```python
from build123d import *

# Parameters (mm, degrees)
SKETCH1_W            = 40
SKETCH1_H            = 20
BOSS_EXTRUDE1_DEPTH  = 35.3
BOSS_EXTRUDE2_DEPTH  = 2
SKETCH3_R            = 6.458580866
BOSS_EXTRUDE3_DEPTH  = 1.5
SKETCH4_R            = 5.433415679
BOSS_EXTRUDE4_DEPTH  = 1.5
SKETCH5_R            = 2.875
BOSS_EXTRUDE5_DEPTH  = 4
SKETCH6_W            = 20
SKETCH6_H            = 2.5
BOSS_EXTRUDE6_DEPTH  = 6
CUT_EXTRUDE1_DEPTH   = 7
SKETCH8_W            = 20
SKETCH8_H            = 2.5
BOSS_EXTRUDE7_DEPTH  = 6
CUT_EXTRUDE2_DEPTH   = 7
SKETCH11_W           = 7
SKETCH11_H           = 4
BOSS_EXTRUDE8_DEPTH  = 6
SKETCH12_W           = 6.5
SKETCH12_H           = 3.5
CUT_EXTRUDE3_DEPTH   = 6
SKETCH13_W           = 6
SKETCH13_H           = 1.3
BOSS_EXTRUDE9_DEPTH  = 1.5
SKETCH14_W           = 6
SKETCH14_H           = 1.3
BOSS_EXTRUDE10_DEPTH = 1.5
CUT_EXTRUDE4_DEPTH   = 1.5
CUT_EXTRUDE5_DEPTH   = 1.5
SKETCH17_R           = 1.5
CUT_EXTRUDE6_DEPTH   = 4


with BuildPart() as part:
    # Sketch1 → Boss-Extrude1 (new body)
    with BuildSketch(Plane(origin=(0, 0, 0), x_dir=(1, 0, 0), z_dir=(0, 1, 0))):
        with Locations((20, 10)):
            Rectangle(SKETCH1_W, SKETCH1_H)
    extrude(amount=BOSS_EXTRUDE1_DEPTH)

    # Sketch2 → Boss-Extrude2 (add)
    with BuildSketch(Plane(origin=(0, 35.3, 0), x_dir=(1, 0, 0), z_dir=(0, 1, 0))):
        with BuildLine():
            Line((34, 5.599382986), (34, 1))
            Line((34, 1), (14.359898944, 1))
            ThreePointArc((14.359898944, 1), (0.001, 10), (14.359898944, 19))
            Line((14.359898944, 19), (34, 19))
            Line((34, 19), (34, 14.400617014))
            ThreePointArc((34, 14.400617014), (36.031185557, 10), (34, 5.599382986))
        make_face()
    extrude(amount=BOSS_EXTRUDE2_DEPTH)

    # Sketch3 → Boss-Extrude3 (add)
    with BuildSketch(Plane(origin=(0, 37.3, 0), x_dir=(1, 0, 0), z_dir=(0, 1, 0))):
        with Locations((9.993186342, 10)):
            Circle(SKETCH3_R)
    extrude(amount=BOSS_EXTRUDE3_DEPTH)

    # Sketch4 → Boss-Extrude4 (add)
    with BuildSketch(Plane(origin=(0, 38.8, 0), x_dir=(1, 0, 0), z_dir=(0, 1, 0))):
        with Locations((9.970242147, 10)):
            Circle(SKETCH4_R)
    extrude(amount=BOSS_EXTRUDE4_DEPTH)

    # Sketch5 → Boss-Extrude5 (add)
    with BuildSketch(Plane(origin=(0, 40.3, 0), x_dir=(1, 0, 0), z_dir=(0, 1, 0))):
        with Locations((9.970242147, 10)):
            Circle(SKETCH5_R)
    extrude(amount=BOSS_EXTRUDE5_DEPTH)

    # Sketch6 → Boss-Extrude6 (add)
    with BuildSketch(Plane(origin=(40, 0, 0), x_dir=(0, 0, -1), z_dir=(1, 0, 0))):
        with Locations((10, 27.55)):
            Rectangle(SKETCH6_W, SKETCH6_H)
    extrude(amount=BOSS_EXTRUDE6_DEPTH)

    # Sketch7 → Cut-Extrude1 (cut)
    with BuildSketch(Plane(origin=(0, 28.8, 0), x_dir=(1, 0, 0), z_dir=(0, 1, 0))):
        with BuildLine():
            ThreePointArc((46, 3.177124344), (46.370828693, 3.792893219), (46.5, 4.5))
            ThreePointArc((46.5, 4.5), (46.370828693, 5.207106781), (46, 5.822875656))
            Line((46, 5.822875656), (46, 3.177124344))
        make_face()
        with BuildLine():
            Line((46, 3.177124344), (46, 5.822875656))
            ThreePointArc((46, 5.822875656), (43.792893219, 6.370828693), (42.5, 4.5))
            ThreePointArc((42.5, 4.5), (43.792893219, 2.629171307), (46, 3.177124344))
        make_face()
        with BuildLine():
            ThreePointArc((42.5, 15.5), (43.792893219, 13.629171307), (46, 14.177124344))
            Line((46, 14.177124344), (46, 16.822875656))
            ThreePointArc((46, 16.822875656), (43.792893219, 17.370828693), (42.5, 15.5))
        make_face()
        with BuildLine():
            Line((46, 16.822875656), (46, 14.177124344))
            ThreePointArc((46, 14.177124344), (46.370828693, 14.792893219), (46.5, 15.5))
            ThreePointArc((46.5, 15.5), (46.370828693, 16.207106781), (46, 16.822875656))
        make_face()
    extrude(amount=-CUT_EXTRUDE1_DEPTH, mode=Mode.SUBTRACT)

    # Sketch8 → Boss-Extrude7 (add)
    with BuildSketch(Plane.ZY):
        with Locations((-10, 27.55)):
            Rectangle(SKETCH8_W, SKETCH8_H)
    extrude(amount=BOSS_EXTRUDE7_DEPTH)

    # Sketch9 → Cut-Extrude2 (cut)
    with BuildSketch(Plane(origin=(0, 28.8, 0), x_dir=(1, 0, 0), z_dir=(0, 1, 0))):
        with BuildLine():
            ThreePointArc((-6, 14.177124344), (-3.792893219, 13.629171307), (-2.5, 15.5))
            ThreePointArc((-2.5, 15.5), (-3.792893219, 17.370828693), (-6, 16.822875656))
            Line((-6, 16.822875656), (-6, 14.177124344))
        make_face()
        with BuildLine():
            Line((-6, 14.177124344), (-6, 16.822875656))
            ThreePointArc((-6, 16.822875656), (-6.5, 15.5), (-6, 14.177124344))
        make_face()
        with BuildLine():
            ThreePointArc((-2.5, 4.5), (-3.792893219, 6.370828693), (-6, 5.822875656))
            Line((-6, 5.822875656), (-6, 3.177124344))
            ThreePointArc((-6, 3.177124344), (-3.792893219, 2.629171307), (-2.5, 4.5))
        make_face()
        with BuildLine():
            Line((-6, 3.177124344), (-6, 5.822875656))
            ThreePointArc((-6, 5.822875656), (-6.5, 4.5), (-6, 3.177124344))
        make_face()
    extrude(amount=-CUT_EXTRUDE2_DEPTH, mode=Mode.SUBTRACT)

    # Sketch11 → Boss-Extrude8 (add)
    with BuildSketch(Plane.ZY):
        with Locations((-10.225128457, 8.7)):
            Rectangle(SKETCH11_W, SKETCH11_H)
    extrude(amount=BOSS_EXTRUDE8_DEPTH)

    # Sketch12 → Cut-Extrude3 (cut)
    with BuildSketch(Plane.ZY.offset(6)):
        with Locations((-10.225128457, 8.7)):
            Rectangle(SKETCH12_W, SKETCH12_H)
    extrude(amount=-CUT_EXTRUDE3_DEPTH, mode=Mode.SUBTRACT)

    # Sketch13 → Boss-Extrude9 (add)
    with BuildSketch(Plane(origin=(0, 28.8, 0), x_dir=(1, 0, 0), z_dir=(0, 1, 0))):
        with Locations((43, 10)):
            Rectangle(SKETCH13_W, SKETCH13_H)
    extrude(amount=BOSS_EXTRUDE9_DEPTH)

    # Sketch14 → Boss-Extrude10 (add)
    with BuildSketch(Plane(origin=(0, 28.8, 0), x_dir=(1, 0, 0), z_dir=(0, 1, 0))):
        with Locations((-3, 10)):
            Rectangle(SKETCH14_W, SKETCH14_H)
    extrude(amount=BOSS_EXTRUDE10_DEPTH)

    # Sketch15 → Cut-Extrude4 (cut)
    with BuildSketch(Plane.XY.offset(-9.35)):
        Polygon((40, 30.3), (46, 28.8), (46, 30.3), align=None)
    extrude(amount=-CUT_EXTRUDE4_DEPTH, mode=Mode.SUBTRACT)

    # Sketch16 → Cut-Extrude5 (cut)
    with BuildSketch(Plane.XY.offset(-9.35)):
        Polygon((-6, 28.8), (-6, 30.3), (0, 30.3), align=None)
    extrude(amount=-CUT_EXTRUDE5_DEPTH, mode=Mode.SUBTRACT)

    # Sketch17 → Cut-Extrude6 (cut)
    with BuildSketch(Plane(origin=(0, 44.3, 0), x_dir=(1, 0, 0), z_dir=(0, 1, 0))):
        with Locations((9.970242147, 10)):
            Circle(SKETCH17_R)
    extrude(amount=-CUT_EXTRUDE6_DEPTH, mode=Mode.SUBTRACT)


solid = part.part
```
For this review, take the finished solid that the model builds, in its own axes (mm). A direction names the side the tool comes from. Coordinates: 2 decimals unless noted, no trailing zeros. Loops run counter-clockwise (first coordinate to the right, second up) from the corner with the lowest first, then second, coordinate; pieces in that order, holes last.
1. Mouldability with a two-part tool opening along Y and no side actions: class faces 4 (the flat face through (-3, 9, -6.975)), 5 (the flat face through (-2.96, 29.56, -9.99)), 6 (the flat face through (-6, 28, -10)) as +Y half, -Y half, draft (parallel to the pull), parting line (faces both ways), or undercut.
2. For line 1 (Y direction, x = -2, z = -9); line 2 (X direction, y = 42.95, z = -10); line 3 (Y direction, x = 17.5, z = -6.25), list the stretches that pass through material, from the lowest coordinate up.
3. Add section B-B, the plane y = 16. Give the boundary of the cut face in (x, z), then the cut area to 3 significant figures.
4. Insertion check: P1, Ø1.5, axis at x = 28, z = -13.5, coming from the +Y side; P2, Ø1.8, axis at x = -2, z = -10, coming from the +Y side (3 decimals); P3, Ø3, axis at x = -2.5, z = -4.5, coming from the +Y side. Each pin has a flat end and moves straight along its axis. Give the tip position at first contact, or say it passes through.
5. Add section A-A, the plane x = 26.5. Give the boundary of the cut face in (y, z).
6. For faces 1 (the flat face through (-2, 28.8, -5)), 2 (the flat face through (24, 36, -1)), 3 (the cylindrical face through (0, 36, -10)), list the 3-axis set-ups (+Z, -Z, +X, -X, +Y, -Y) from which the entire face can be reached by the end or side of a thin tool; tool diameter is ignored.
Result:
1. face 4: undercut
1. face 5: +Y half
1. face 6: draft
2. line 1: y = 6.7 to 6.95, 10.45 to 10.7, 26.3 to 28.8
2. line 2: x = 7.1 to 8.47, 11.47 to 12.85
2. line 3: y = 0 to 37.3
3. outline: (0, -20) - (40, -20) - (40, 0) - (0, 0) - close
3. area: 800 mm2
4. P1: stops at y = 37.3
4. P2: stops at y = 30.025
4. P3: stops at y = 28.8
5. outline: (0, -20) - (35.3, -20) - (35.3, -19) - (37.3, -19) - (37.3, -1) - (35.3, -1) - (35.3, 0) - (0, 0) - close
6. face 1: +Z, -X, +Y
6. face 2: +Z, +X, +Y
6. face 3: +Y
